```python
from build123d import *

# Parameters (mm, degrees)
EXTRUDE_1_DEPTH     = 25
CUT_EXTRUDE_1_DEPTH = 25
SKETCH_3_R          = 1.6
CUT_EXTRUDE_2_DEPTH = 2
SKETCH_4_R          = 5
CUT_EXTRUDE_3_DEPTH = 25


with BuildPart() as part:
    # 草图1 → 凸台-拉伸1 (new, symmetric)
    with BuildSketch(Plane.XY):
        Polygon((0, 0), (-25, 0), (-25, 50), (25, 50), (25, 0), align=None)
    extrude(amount=EXTRUDE_1_DEPTH, both=True)

    # 草图2 → 切除-拉伸1 (cut, symmetric)
    with BuildSketch(Plane.XY):
        with BuildLine():
            Line((-25, 50), (-20, 50))
            Line((-20, 50), (-20, 2.5))
            ThreePointArc((-20, 2.5), (-20.146446609, 2.146446609), (-20.5, 2))
            Line((-20.5, 2), (-25, 2))
            Line((-25, 2), (-25, 50))
        make_face()
        with BuildLine():
            Line((25, 50), (20, 50))
            Line((20, 50), (20, 2.5))
            ThreePointArc((20, 2.5), (20.146446609, 2.146446609), (20.5, 2))
            Line((20.5, 2), (25, 2))
            Line((25, 2), (25, 50))
        make_face()
        with BuildLine():
            Line((-16.5, 0), (16.5, 0))
            Line((16.5, 0), (16.5, 47.5))
            ThreePointArc((16.5, 47.5), (16.353553391, 47.853553391), (16, 48))
            Line((16, 48), (-16, 48))
            ThreePointArc((-16, 48), (-16.353553391, 47.853553391), (-16.5, 47.5))
            Line((-16.5, 47.5), (-16.5, 0))
        make_face()
    extrude(amount=CUT_EXTRUDE_1_DEPTH, both=True, mode=Mode.SUBTRACT)

    # 草图3 → 切除-拉伸2 (cut)
    with BuildSketch(Plane(origin=(0, 50, 0), x_dir=(1, 0, 0), z_dir=(0, 1, 0))):
        with Locations(Location((0, 4, 0), (0, 0, 270))):
            Circle(SKETCH_3_R)
        with Locations(Location((0, -4, 0), (0, 0, 270))):
            Circle(SKETCH_3_R)
        with BuildLine():
            Line((3, 7.5), (14.5, 7.5))
            ThreePointArc((14.5, 7.5), (14.853553391, 7.353553391), (15, 7))
            Line((15, 7), (15, -7))
            ThreePointArc((15, -7), (14.853553391, -7.353553391), (14.5, -7.5))
            Line((14.5, -7.5), (3, -7.5))
            ThreePointArc((3, -7.5), (2.646446609, -7.353553391), (2.5, -7))
            Line((2.5, -7), (2.5, 7))
            ThreePointArc((2.5, 7), (2.646446609, 7.353553391), (3, 7.5))
        make_face()
        with BuildLine():
            Line((-14.5, 7.5), (-3, 7.5))
            ThreePointArc((-3, 7.5), (-2.646446609, 7.353553391), (-2.5, 7))
            Line((-2.5, 7), (-2.5, 0))
            Line((-2.5, 0), (-2.5, -7))
            ThreePointArc((-2.5, -7), (-2.646446609, -7.353553391), (-3, -7.5))
            Line((-3, -7.5), (-14.5, -7.5))
            ThreePointArc((-14.5, -7.5), (-14.853553391, -7.353553391), (-15, -7))
            Line((-15, -7), (-15, 7))
            ThreePointArc((-15, 7), (-14.853553391, 7.353553391), (-14.5, 7.5))
        make_face()
    extrude(amount=-CUT_EXTRUDE_2_DEPTH, mode=Mode.SUBTRACT)

    # 草图4 → 切除-拉伸3 (cut, symmetric)
    with BuildSketch(Plane(origin=(0, 0, 0), x_dir=(0, 0, -1), z_dir=(1, 0, 0))):
        with Locations((0, 35)):
            Circle(SKETCH_4_R)
    extrude(amount=CUT_EXTRUDE_3_DEPTH, both=True, mode=Mode.SUBTRACT)


solid = part.part
```
Check sheet for the modelled part. Datum: model origin and axes. Units: mm. A direction names the side the tool comes from. Give positions to 0.01 mm unless a question says otherwise; leave off trailing zeros. Write each loop counter-clockwise with the first axis right and the second up, starting at its lowest first coordinate (ties: lowest second). Pieces come first, ordered by that corner, then holes.
Item 1: Gauge pin test, flat ends, axial feed: pin 1 (1.6 mm diameter, centred on y = 49, z = 2.5, fed in from -X); pin 2 (24 mm diameter, centred on y = 12, z = -6.5, fed in from +X); pin 3 (5 mm diameter, centred on x = -9, z = 15, fed in from -Y); pin 4 (0.6 mm diameter, centred on y = 49.5, z = 3.5, fed in from +X). Record the tip position at first contact, or that the pin passes through.
Item 2: Cross-section at A-A (y = 9). Enter the section's corners in (x, z).
Item 3: Access from +Z, -Z, +X, -X, +Y, -Y to the whole of each face (thin tool, end or side, straight path). Record for faces 1 (the face through (-20, 27, 0)), 2 (the face through (16.5, 23, 0)), 3 (the face through (9, 49, 7.5)).
Item 4: Draft check along Y on faces 4 (the face through (17, 29, 25)), 5 (the face through (23, 2, 0)), 6 (the face through (18, 39, -3)). Enter one of: released by +Y, released by -Y, zero draft, split by the parting line, or undercut.
Item 5: Cross-section at D-D (z = -20.5). Enter the section's corners in (x, y).
Item 6: Cross-section at B-B (x = 0). Enter the section's corners in (y, z), and give its area (3 significant figures).
Item 7: Cross-section at C-C (y = 35). Enter the section's corners in (x, z).
Item 8: Scan lines: L1, parallel to X at y = 49.1, z = 4; L2, parallel to X at y = 14, z = 22; L3, parallel to Y at x = -18.25, z = 0. Record each from-to range of solid material in increasing order.
Report:
1. pin 1: stops at x = -20
1. pin 2: stops at x = 25
1. pin 3: stops at y = 48
1. pin 4: stops at x = 20
2. outline: (-20, -25) - (-16.5, -25) - (-16.5, 25) - (-20, 25) - close; (16.5, -25) - (20, -25) - (20, 25) - (16.5, 25) - close
3. face 1: +Z, -Z, -X, +Y
3. face 2: +Z, -Z, -Y
3. face 3: +Y, -Y
4. face 4: zero draft
4. face 5: released by +Y
4. face 6: undercut
5. outline: (-25, 0) - (-16.5, 0) - (-16.5, 47.5) arc R0.5 cw to (-16, 48) - (16, 48) arc R0.5 cw to (16.5, 47.5) - (16.5, 0) - (25, 0) - (25, 2) - (20.5, 2) arc R0.5 cw to (20, 2.5) - (20, 50) - (-20, 50) - (-20, 2.5) arc R0.5 cw to (-20.5, 2) - (-25, 2) - close
6. outline: (48, -25) - (50, -25) - (50, -5.6) - (48, -5.6) - close; (48, -2.4) - (50, -2.4) - (50, 2.4) - (48, 2.4) - close; (48, 5.6) - (50, 5.6) - (50, 25) - (48, 25) - close
6. area: 87.2 mm2
7. outline: (-20, -25) - (-16.5, -25) - (-16.5, -5) - (-20, -5) - close; (-20, 5) - (-16.5, 5) - (-16.5, 25) - (-20, 25) - close; (16.5, -25) - (20, -25) - (20, -5) - (16.5, -5) - close; (16.5, 5) - (20, 5) - (20, 25) - (16.5, 25) - close
8. L1: x = -20 to -15, -2.5 to -1.6, 1.6 to 2.5, 15 to 20
8. L2: x = -20 to -16.5, 16.5 to 20
8. L3: y = 0 to 30, 40 to 50
